Read the model definition and answer for the solid it produces. Units are mm, in the model's axes. Round coordinates to 2 decimals unless told otherwise and drop trailing zeros. Answer as a JSON object with one key per item and string values. Group by question number.
Q1. Consider line 1 (Z direction, x = -60, y = -2.2); line 2 (Z direction, x = 21, y = -3.9); line 3 (Z direction, x = -17.5, y = -2). Determine where each line is inside the solid, lowest interval first.
Q2. A cutting plane is placed at A-A on y = -3.7. Count the separate pieces of the cut face and the enclosed holes in it, and give its area (3 significant figures).
Q3. Given pin 1 Ø11.5 at (x, z) = (-59.32, 60.22) entering from +Y; pin 2 Ø5.5 at (x, z) = (21.48, 118.17) entering from -Y, each flat-ended and moving along its own axis, determine where each tip first touches the part or whether it passes through.
Q4. The mould has two halves that part along X. Classify faces 1 (the cylindrical face through (-63.12, -2.37, -58.1)), 2 (the cylindrical face through (-68.19, -2.37, -123.65)), 3 (the cylindrical face through (68.19, -2.37, 123.65)): pulls with the +X half, pulls with the -X half, needs draft (parallel to the pull), parting line crosses it, or undercut.
```python
from build123d import *

# Parameters (mm, degrees)
ESBO_O1_R          = 4.5
FLANGE_BASE1_DEPTH = 4.8


# Sheet-metal steps are written as plain solids
with BuildPart() as part:
    # Esboço1 → Flange-base1 (new body)
    with BuildSketch(Plane(origin=(0, 0, 0), x_dir=(1, 0, 0), z_dir=(0, 1, 0))):
        with BuildLine():
            Line((-61.2, -126.5), (61.2, -126.5))
            ThreePointArc((61.2, -126.5), (68.271067812, -123.571067812), (71.2, -116.5))
            Line((71.2, -116.5), (71.2, 116.5))
            ThreePointArc((71.2, 116.5), (68.271067812, 123.571067812), (61.2, 126.5))
            Line((61.2, 126.5), (-61.2, 126.5))
            ThreePointArc((-61.2, 126.5), (-68.271067812, 123.571067812), (-71.2, 116.5))
            Line((-71.2, 116.5), (-71.2, -116.5))
            ThreePointArc((-71.2, -116.5), (-68.271067812, -123.571067812), (-61.2, -126.5))
        make_face()
        with Locations(Location((-59.32366364, 113.632351832, 0), (0, 0, 270))):
            Circle(ESBO_O1_R, mode=Mode.SUBTRACT)
        with Locations(Location((61.87633636, 113.632351832, 0), (0, 0, 270))):
            Circle(ESBO_O1_R, mode=Mode.SUBTRACT)
        with Locations(Location((-59.32366364, -118.167648168, 0), (0, 0, 270))):
            Circle(ESBO_O1_R, mode=Mode.SUBTRACT)
        with Locations(Location((61.87633636, -118.167648168, 0), (0, 0, 270))):
            Circle(ESBO_O1_R, mode=Mode.SUBTRACT)
        with Locations(Location((-18.92366364, 113.632351832, 0), (0, 0, 270))):
            Circle(ESBO_O1_R, mode=Mode.SUBTRACT)
        with Locations(Location((21.47633636, 113.632351832, 0), (0, 0, 270))):
            Circle(ESBO_O1_R, mode=Mode.SUBTRACT)
        with Locations(Location((61.87633636, 55.682351832, 0), (0, 0, 270))):
            Circle(ESBO_O1_R, mode=Mode.SUBTRACT)
        with Locations(Location((61.87633636, -2.267648168, 0), (0, 0, 270))):
            Circle(ESBO_O1_R, mode=Mode.SUBTRACT)
        with Locations(Location((61.87633636, -60.217648168, 0), (0, 0, 270))):
            Circle(ESBO_O1_R, mode=Mode.SUBTRACT)
        with Locations(Location((21.47633636, -118.167648168, 0), (0, 0, 90))):
            Circle(ESBO_O1_R, mode=Mode.SUBTRACT)
        with Locations(Location((-18.92366364, -118.167648168, 0), (0, 0, 90))):
            Circle(ESBO_O1_R, mode=Mode.SUBTRACT)
        with Locations(Location((-59.32366364, -60.217648168, 0), (0, 0, 90))):
            Circle(ESBO_O1_R, mode=Mode.SUBTRACT)
        with Locations(Location((-59.32366364, -2.267648168, 0), (0, 0, 90))):
            Circle(ESBO_O1_R, mode=Mode.SUBTRACT)
        with Locations(Location((-59.32366364, 55.682351832, 0), (0, 0, 90))):
            Circle(ESBO_O1_R, mode=Mode.SUBTRACT)
    extrude(amount=-FLANGE_BASE1_DEPTH)


solid = part.part
```
Result set:
{
 "1": {"line 1": "z = -126.5 to -118.08, -109.18 to -60.13, -51.23 to -2.18, 6.72 to 55.77, 64.67 to 113.72, 122.62 to 126.5", "line 2": "z = -126.5 to -118.11, -109.16 to 113.69, 122.64 to 126.5", "line 3": "z = -126.5 to -117.9, -109.36 to 113.9, 122.44 to 126.5"},
 "2": {"separate pieces": "1", "enclosed holes": "14", "area": "35,100 mm²"},
 "3": {"pin 1": "stops at y = 0", "pin 2": "passes through"},
 "4": {"face 1": "undercut", "face 2": "pulls with the -X half", "face 3": "pulls with the +X half"}
}
